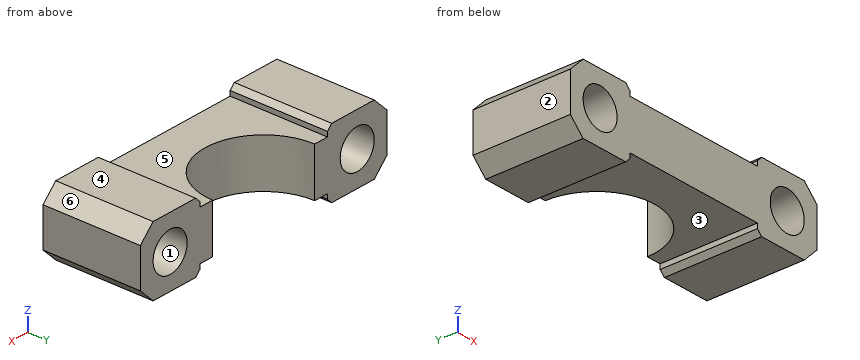
```python
from build123d import *

# Parameters (mm, degrees)
SKETCH_R        = 2
PAD_DEPTH       = 10
POCKET_DEPTH    = 6.001
CHAMFER_SIZE    = 1.5
CHAMFER001_SIZE = 0.5


with BuildPart() as part:
    # Sketch → Pad (new body)
    with BuildSketch(Plane.XZ):
        Polygon((0, 7), (0, 0), (7, 0), (7, 1), (22, 1), (22, 0), (29, 0), (29, 7), (22, 7), (22, 6), (7, 6), (7, 7), align=None)
        with Locations((3.5, 3.5)):
            Circle(SKETCH_R, mode=Mode.SUBTRACT)
        with Locations((25.5, 3.5)):
            Circle(SKETCH_R, mode=Mode.SUBTRACT)
    extrude(amount=PAD_DEPTH)

    # Sketch001 (on Face10 of Pad) → Pocket (cut, through all)
    with BuildSketch(Plane(origin=(0, 0, 6), x_dir=(-1, 0, 0), z_dir=(0, 0, 1))):
        with BuildLine():
            ThreePointArc((-8.5, 0), (-14.5, 6), (-20.5, 0))
            Line((-20.5, 0), (-8.5, 0))
        make_face()
    extrude(amount=-POCKET_DEPTH, mode=Mode.SUBTRACT)

    # Chamfer
    chamfer_edges = [part.edges().sort_by_distance(p)[0] for p in [
        (0, -5, 0),
        (0, -5, 7),
        (29, -5, 0),
        (29, -5, 7),
    ]]
    chamfer(chamfer_edges, length=CHAMFER_SIZE)

    # Chamfer001
    chamfer001_edges = [part.edges().sort_by_distance(p)[0] for p in [
        (7, -5, 7),
        (22, -5, 7),
        (7, -5, 0),
        (22, -5, 0),
    ]]
    chamfer(chamfer001_edges, length=CHAMFER001_SIZE)


solid = part.part
```
Can you work these out from the model? Positions are in its coordinate system, mm. Face numbers are marked on the shaded views. A direction names the side the tool comes from. Round coordinates to 2 decimals unless told otherwise and drop trailing zeros. Loops run counter-clockwise (first coordinate to the right, second up) from the corner with the lowest first, then second, coordinate; pieces in that order, holes last. Notation, with made-up numbers: M 89.5,47.25 L 99.5,47.25 A18 cw 99.5,71.25 Z; hole C 4.25,7 d7. An arc over 180 degrees is marked long. Answer as a JSON object with one key per item and string values. Group by question number.
Q1. Will these pins go through, and if not, where does the flat tip stop? pin 1 (0.6 mm diameter, centred on y = -4, z = 6.5, fed in from -X); pin 2 (3 mm diameter, centred on x = 13.5, y = -2.5, fed in from -Z); pin 3 (0.6 mm diameter, centred on y = -3.5, z = 6, fed in from +X); pin 4 (4 mm diameter, centred on x = 19.5, y = -1.5, fed in from -Z).
Q2. On a 3-axis mill with a long thin cutter (end or side, diameter ignored), from which of +Z, -Z, +X, -X, +Y, -Y can I reach the whole of each face in a straight line? I mean the marked faces 5 and 6. Say none if no direction works.
Q3. Please list where these lines run through material, in increasing order: L1, parallel to Z at x = 3.5, y = -3.75; L2, parallel to X at y = -3, z = 2; L3, parallel to Z at x = 16, y = -9.25.
Q4. Imagine slicing it at D-D, the plane y = -6.5. Please give me the cut outline in (x, z).
Q5. We'd pull the mould along X, two halves only. Please class the marked faces 1, 2, 3 and 4: +X half, -X half, draft (parallel to the pull), parting line (faces both ways), or undercut.
Q6. Imagine slicing it at A-A, the plane z = 3.5. Please give me the cut outline in (x, y).
Q7. Imagine slicing it at B-B, the plane y = -2.75. Please give me the cut outline in (x, z).
Q8. Imagine slicing it at C-C, the plane x = 3.5. Please give me the cut outline in (y, z).
Findings:
{
 "1": {"pin 1": "stops at x = 0.7", "pin 2": "passes through", "pin 3": "stops at x = 28.8", "pin 4": "stops at z = 1"},
 "2": {"face 5": "+Z, +Y, -Y", "face 6": "+Z, +X, +Y, -Y"},
 "3": {"L1": "z = 0 to 1.5, 5.5 to 7", "L2": "x = 0 to 2.18, 4.82 to 9.3, 19.7 to 24.18, 26.82 to 29", "L3": "z = 1 to 6"},
 "4": {"outline": "M 0,1.5 L 1.5,0 L 6.5,0 L 7,0.5 L 7,1 L 22,1 L 22,0.5 L 22.5,0 L 27.5,0 L 29,1.5 L 29,5.5 L 27.5,7 L 22.5,7 L 22,6.5 L 22,6 L 7,6 L 7,6.5 L 6.5,7 L 1.5,7 L 0,5.5 Z; hole C 3.5,3.5 d4; hole C 25.5,3.5 d4"},
 "5": {"face 1": "undercut", "face 2": "-X half", "face 3": "undercut", "face 4": "draft"},
 "6": {"outline": "M 0,-10 L 1.5,-10 L 1.5,0 L 0,0 Z; M 5.5,-10 L 23.5,-10 L 23.5,0 L 20.5,0 A6 cw 8.5,0 L 5.5,0 Z; M 27.5,-10 L 29,-10 L 29,0 L 27.5,0 Z"},
 "7": {"outline": "M 0,1.5 L 1.5,0 L 6.5,0 L 7,0.5 L 7,1 L 9.17,1 L 9.17,6 L 7,6 L 7,6.5 L 6.5,7 L 1.5,7 L 0,5.5 Z; M 19.83,1 L 22,1 L 22,0.5 L 22.5,0 L 27.5,0 L 29,1.5 L 29,5.5 L 27.5,7 L 22.5,7 L 22,6.5 L 22,6 L 19.83,6 Z; hole C 3.5,3.5 d4; hole C 25.5,3.5 d4"},
 "8": {"outline": "M -10,0 L 0,0 L 0,1.5 L -10,1.5 Z; M -10,5.5 L 0,5.5 L 0,7 L -10,7 Z"}
}
